```python
from build123d import *

# Parameters (mm, degrees)
BOSS_EXTRUDE1_DEPTH = 3
FILLET1_R           = 5
FILLET2_R           = 2.5
FILLET3_R           = 1


with BuildPart() as part:
    # Sketch1 → Boss-Extrude1 (new body)
    with BuildSketch(Plane(origin=(0, 0, 0), x_dir=(1, 0, 0), z_dir=(0, 1, 0))):
        with BuildLine():
            Line((-62.418566214, -50.1586621), (-58.418566214, -50.1586621))
            Line((-58.418566214, -50.1586621), (-58.418566214, -38.1586621))
            Line((-58.418566214, -38.1586621), (-48.418566214, -38.1586621))
            Line((-48.418566214, -38.1586621), (-48.418566214, -50.1586621))
            Line((-48.418566214, -50.1586621), (-44.418566214, -50.1586621))
            Line((-44.418566214, -50.1586621), (-43.418817081, -60.156153425))
            Line((-43.418817081, -60.156153425), (-43.418817081, -62.1586621))
            Line((-43.418817081, -62.1586621), (-40.418817081, -62.1586621))
            Line((-40.418817081, -62.1586621), (-40.418817081, -60.1586621))
            Line((-40.418817081, -60.1586621), (-38.682853905, -54.924562388))
            ThreePointArc((-38.682853905, -54.924562388), (-37.311808452, -53.840242209), (-35.772499384, -54.668519625))
            Line((-35.772499384, -54.668519625), (-32.803457275, -60.1586621))
            Line((-32.803457275, -60.1586621), (28.581433786, -60.1586621))
            Line((28.581433786, -60.1586621), (28.581433786, -62.1586621))
            Line((28.581433786, -62.1586621), (31.581433786, -62.1586621))
            Line((31.581433786, -62.1586621), (31.581433786, -60.208800497))
            Line((31.581433786, -60.208800497), (32.581433786, -50.211334262))
            Line((32.581433786, -50.211334262), (36.581433786, -50.211334262))
            Line((36.581433786, -50.211334262), (36.581433786, -38.211334262))
            Line((36.581433786, -38.211334262), (46.581433786, -38.211334262))
            Line((46.581433786, -38.211334262), (46.581433786, -50.211334262))
            Line((46.581433786, -50.211334262), (50.581433786, -50.211334262))
            Line((50.581433786, -50.211334262), (41.830582941, -65.1586621))
            Line((41.830582941, -65.1586621), (-53.758312176, -65.1586621))
            Line((-53.758312176, -65.1586621), (-62.202371167, -60.610709304))
            ThreePointArc((-62.202371167, -60.610709304), (-62.450096964, -60.048239346), (-61.965274707, -59.670498822))
            Line((-61.965274707, -59.670498822), (-59.524980934, -59.670498822))
            ThreePointArc((-59.524980934, -59.670498822), (-58.225942828, -58.920498822), (-58.225942828, -57.420498822))
            Line((-58.225942828, -57.420498822), (-62.418566214, -50.1586621))
        make_face()
        Polygon((36.547763078, -54.211334262), (39.581433786, -54.211334262), (39.581433786, -44.211334262), (39.581433786, -41.211334262), (43.581433786, -41.211334262), (43.581433786, -44.211334262), (43.604572315, -54.211334262), (40.093380681, -60.208800497), (35.947864455, -60.208800497), align=None, mode=Mode.SUBTRACT)
        Polygon((-55.418566214, -41.1586621), (-51.418566214, -41.1586621), (-51.418566214, -44.1586621), (-51.418566214, -54.1586621), (-48.038516462, -54.1586621), (-47.438516462, -60.1586621), (-52.026261368, -60.1586621), (-55.490362984, -54.1586621), (-55.418566214, -44.1586621), align=None, mode=Mode.SUBTRACT)
    extrude(amount=BOSS_EXTRUDE1_DEPTH)

    # Fillet1
    fillet1_edges = [part.edges().sort_by_distance(p)[0] for p in [
        (41.830582941, 1.5, 65.1586621),
        (-53.758312176, 1.5, 65.1586621),
    ]]
    fillet(fillet1_edges, radius=FILLET1_R)

    # Fillet2
    fillet2_edges = [part.edges().sort_by_distance(p)[0] for p in [
        (-58.418566214, 1.5, 38.1586621),
        (-48.418566214, 1.5, 38.1586621),
        (36.581433786, 1.5, 38.211334262),
        (46.581433786, 1.5, 38.211334262),
    ]]
    fillet(fillet2_edges, radius=FILLET2_R)

    # Fillet3
    fillet3_edges = [part.edges().sort_by_distance(p)[0] for p in [
        (-32.803457275, 1.5, 60.1586621),
    ]]
    fillet(fillet3_edges, radius=FILLET3_R)


solid = part.part
```
The model under review builds one solid part; all positions refer to its coordinate system, in mm. A direction names the side the tool comes from. Coordinates: 2 decimals unless noted, no trailing zeros. Order: outer loops, then holes, each group sorted by start corner. A loop starts at its lowest first (then second) coordinate and runs counter-clockwise, first axis right, second up. Notation, with made-up numbers: (7.5, 62.5) -> (65.5, 62.5) arc R3 cw to (65.5, 67.5) -> close; hole circle Ø7 at (-12, 12.25). An arc over 180 degrees is marked (long way). Answer in a Markdown table with one row per item. Add a question column.
Item 1: We need section A-A on z = 58.5. Write out the cut boundary in (x, y).
Item 2: To check wall thickness, follow probe 1 along X at (y, z) = (1.45, 42.25); probe 2 along Z at (x, y) = (39, 2.25); probe 3 along X at (y, z) = (1, 62). State the ranges of each line that lie inside material, in increasing order.
Item 3: Machinability: for faces 4 (the flat face through (-2, 1, 60.159)), 5 (the flat face through (-53.734, 1.479, 57.201)), which of the approach directions +Z, -Z, +X, -X, +Y, -Y give a long, thin tool a straight path to every point of the face, cutting with its end or side? Answer none if there is none.
Item 4: We need section C-C on y = 1.6. Give the number of separate pieces and of enclosed holes in the cut face, plus the area to 3 significant figures.
Item 5: We need section D-D on x = -7. Write out the cut boundary in (y, z), plus the area to 3 significant figures.
Item 6: Mouldability with a two-part tool opening along X and no side actions: class faces 1 (the flat face through (-58.419, 1, 45)), 2 (the flat face through (36.581, 1, 46)), 3 (the cylindrical face through (45.869, 1.521, 38.963)) as +X half, -X half, draft (parallel to the pull), parting line (faces both ways), or undercut.
Item 7: Clearance check with flat-ended pins moving along their axes: pin 1 (1.5 mm diameter, centred on x = 37, y = 1.5, fed in from -Z); pin 2 (1 mm diameter, centred on y = 2, z = 61.5, fed in from +X); pin 3 (1.5 mm diameter, centred on x = -31.5, y = 0.5, fed in from -Z). State where each tip first meets the part, or that it passes through.
Item 8: We need section B-B on z = 46. Write out the cut boundary in (x, y).
Final values:
| question | item | result |
|---|---|---|
| 1 | outline | (-58.06, 0) -> (-52.98, 0) -> (-52.98, 3) -> (-58.06, 3) -> close; (-47.6, 0) -> (-43.58, 0) -> (-43.58, 3) -> (-47.6, 3) -> close; (-39.87, 0) -> (-33.7, 0) -> (-33.7, 3) -> (-39.87, 3) -> close; (31.75, 0) -> (36.12, 0) -> (36.12, 3) -> (31.75, 3) -> close; (41.09, 0) -> (45.73, 0) -> (45.73, 3) -> (41.09, 3) -> close |
| 2 | probe 1 | x = -58.42 to -55.42, -51.42 to -48.42, 36.58 to 39.58, 43.58 to 46.58 |
| 2 | probe 2 | z = 38.21 to 54.21, 60.21 to 65.16 |
| 2 | probe 3 | x = -59.62 to -43.42, -40.42 to 28.58, 31.58 to 43.68 |
| 3 | face 4 | -Z, +Y, -Y |
| 3 | face 5 | +Y, -Y |
| 4 | separate pieces | 1 |
| 4 | enclosed holes | 2 |
| 4 | area | 901 mm2 |
| 5 | outline | (0, 60.16) -> (3, 60.16) -> (3, 65.16) -> (0, 65.16) -> close |
| 5 | area | 15.0 mm2 |
| 6 | face 1 | -X half |
| 6 | face 2 | undercut |
| 6 | face 3 | +X half |
| 7 | pin 1 | stops at z = 38.6 |
| 7 | pin 2 | stops at x = 44.27 |
| 7 | pin 3 | stops at z = 60.16 |
| 8 | outline | (-58.42, 0) -> (-55.43, 0) -> (-55.43, 3) -> (-58.42, 3) -> close; (-51.42, 0) -> (-48.42, 0) -> (-48.42, 3) -> (-51.42, 3) -> close; (36.58, 0) -> (39.58, 0) -> (39.58, 3) -> (36.58, 3) -> close; (43.59, 0) -> (46.58, 0) -> (46.58, 3) -> (43.59, 3) -> close |
